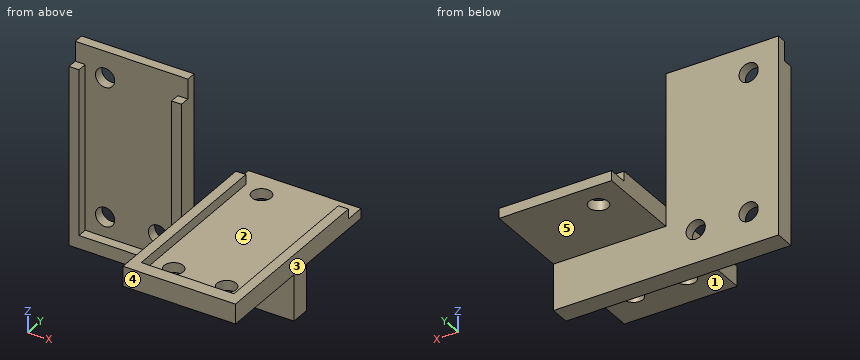
Autodesk Inventor part; units mm, degrees
ref_plane "YZ Plane" through (0, 0, 0) normal (1, 0, 0) x (0, 1, 0)
ref_plane "XZ Plane" through (0, 0, 0) normal (0, 1, 0) x (-1, 0, 0)
ref_plane "XY Plane" through (0, 0, 0) normal (0, 0, 1) x (1, 0, 0)
sketch "Sketch1" plane through (0, 0, 0) normal (0, 0, 1) x (1, 0, 0)
  line L0 (-34, 17) -> (-17, 17)
  line L1 (-17, 17) -> (-17, 30)
  line L2 (-17, 30) -> (0, 30)
  line L3 (0, 30) -> (0, 0)
  line L4 (0, 0) -> (-17, 0)
  line L5 (-17, 0) -> (-17, 14)
  line L6 (-17, 14) -> (-34, 14)
  line L7 (-34, 14) -> (-34, 17)
  dimension "d0" = 17
  dimension "d1" = 13
  dimension "d2" = 17
  dimension "d4" = 17
  dimension "d5" = 14
  dimension "d72" = 3
extrude "Extrusion1" add sketch "Sketch1" along normal blind 30
sketch "Sketch4" plane through (0, 0, 0) normal (0, 0, -1) x (-1, 0, 0)
  line L0 (34, 17) -> (17, 17)
  line L1 (17, 17) -> (17, 30)
  line L2 (17, 30) -> (0, 30)
  line L3 (0, 30) -> (0, 0)
  line L4 (0, 0) -> (17, 0)
  line L5 (17, 0) -> (17, 14)
  line L6 (17, 14) -> (34, 14)
  line L7 (34, 14) -> (34, 17)
  line L8 (17, 0) -> (0, 0)
  line L9 (0, 0) -> (0, 30)
  line L10 (0, 30) -> (17, 30)
  line L11 (17, 30) -> (17, 0)
extrude "Extrusion4" cut sketch "Sketch4" against normal blind 7 contours L11 L5 L4 L3 L2 L1
sketch "Sketch8" plane through (0, 0, 30) normal (0, 0, 1) x (1, 0, 0)
  line L0 (-17, 17) -> (-34, 17)
  line L1 (-34, 17) -> (-34, 14)
  line L2 (-34, 14) -> (-17, 14)
  line L3 (-17, 14) -> (-17, 0)
  line L4 (-17, 0) -> (0, 0)
  line L5 (0, 0) -> (0, 30)
  line L6 (0, 30) -> (-17, 30)
  line L7 (-17, 30) -> (-17, 17)
  line L8 (-17, 30) -> (0, 30)
  line L9 (0, 30) -> (0, 0)
  line L10 (0, 0) -> (-17, 0)
  line L11 (-17, 0) -> (-17, 30)
extrude "Extrusion8" cut sketch "Sketch8" against normal blind 20 contours L7 L6 L5 L4 L3 L11
sketch "Sketch9" plane through (-34, 14, 0) normal (0, -1, 0) x (1, 0, 0)
  line L0 (17, 0) -> (0, 0)
  line L1 (17, 0) -> (17, 7)
  line L2 (17, 7) -> (17, 10)
  line L3 (17, 10) -> (17, 30)
  line L4 (0, 30) -> (17, 30)
  line L5 (0, 0) -> (0, 30)
  line L6 (0, 0) -> (17, 0)
  line L7 (0, 30) -> (17, 30)
  line L8 (17, 0) -> (0, 0)
  line L9 (17, 10) -> (17, 30)
  line L10 (17, 30) -> (0, 30)
  line L11 (0, 0) -> (0, 30)
  line L12 (0, 27) -> (1.5, 27)
  line L13 (1.5, 27) -> (1.5, 2)
  line L14 (1.5, 2) -> (15.5, 2)
  line L15 (17, 27) -> (15.5, 27)
  line L16 (15.5, 27) -> (15.5, 2)
  line L17 (0, 27) -> (0, 30)
  line L18 (17, 30) -> (17, 27)
  point P0 (34, 0)
  dimension "d80" = 1.5
  dimension "d81" = 2
  dimension "d82" = 25
  dimension "d83" = 14
extrude "Extrusion14" cut sketch "Sketch9" against normal blind 1.5 contours L5 L4 L3 L15 L16 L14 L13 L12
sketch "Sketch14" plane through (0, 0, 10) normal (0, 0, 1) x (1, 0, 0)
  line L0 (0, 30) -> (0, 0)
  line L1 (-17, 30) -> (0, 30)
  line L2 (-17, 17) -> (-17, 30)
  line L3 (-17, 14) -> (-17, 17)
  line L4 (-17, 0) -> (-17, 14)
  line L5 (0, 0) -> (-17, 0)
  line L6 (-17, 30) -> (-17, 27)
  line L7 (-17, 30) -> (-17, 17)
  line L8 (-15.5, 27) -> (-15.5, 2)
  line L9 (-15.5, 2) -> (-1.5, 2)
  line L10 (-15.5, 27) -> (-17, 27)
  line L11 (-17, 30) -> (0, 30)
  line L12 (0, 30) -> (-17, 30)
  line L13 (-17, 0) -> (0, 0)
  line L14 (0, 27) -> (0, 30)
  line L15 (-1.5, 27) -> (-1.5, 2)
  line L16 (-1.5, 27) -> (0, 27)
  line L17 (0, 30) -> (0, 0)
  point P0 (0, 30)
  point P1 (-16.25, 27)
  point P2 (-0.75, 27)
  dimension "d87" = 1.5
  dimension "d88" = 2
  dimension "d89" = 25
  dimension "d91" = 1.5
  dimension "d93" = 14
extrude "Extrusion15" cut sketch "Sketch14" against normal blind 1.5 contours L0 L16 L15 L9 L8 L10 L2 L1
sketch "Sketch15" plane through (-34, 15.5, 0) normal (0, -1, 0) x (1, 0, 0)
  line L0 (0, 30) -> (17, 30)
  line L1 (0, 27) -> (0, 30)
  line L2 (1.5, 27) -> (0, 27)
  line L3 (1.5, 2) -> (1.5, 27)
  line L4 (15.5, 2) -> (1.5, 2)
  line L5 (15.5, 27) -> (15.5, 2)
  line L6 (17, 27) -> (15.5, 27)
  line L7 (17, 30) -> (17, 27)
  circle A0 centre (4.5, 26) radius 1.45
  circle A1 centre (4.5, 5) radius 1.45
  circle A2 centre (12.5, 5) radius 1.45
  point P0 (34, 0)
  dimension "d96" = 2.9
  dimension "d97" = 21
  dimension "d98" = 8
  dimension "d99" = 3
  dimension "d100" = 3
extrude "Extrusion16" cut sketch "Sketch15" against normal through all contours A0 | A1 | A2
sketch "Sketch16" plane through (0, 0, 8.5) normal (0, 0, 1) x (1, 0, 0)
  line L0 (-17, 27) -> (-17, 30)
  line L1 (-15.5, 27) -> (-17, 27)
  line L2 (-15.5, 2) -> (-15.5, 27)
  line L3 (-1.5, 2) -> (-15.5, 2)
  line L4 (-1.5, 27) -> (-1.5, 2)
  line L5 (0, 27) -> (-1.5, 27)
  line L6 (0, 30) -> (0, 27)
  line L7 (-17, 30) -> (0, 30)
  circle A0 centre (-12.5, 5) radius 1.45
  circle A1 centre (-4.5, 5) radius 1.45
  circle A2 centre (-12.5, 26) radius 1.45
  point P0 (0, 0)
  dimension "d103" = 3
  dimension "d104" = 3
  dimension "d105" = 8
  dimension "d106" = 21
  dimension "d107" = 2.9
extrude "Extrusion18" cut sketch "Sketch16" against normal through all contours A0 | A1 | A2
sketch "Sketch17" plane through (-17, 14, 0) normal (1, 0, 0) x (0, 0, -1)
  line L0 (0, 0) -> (-7, 0)
  line L1 (0, 3) -> (0, 0)
  line L2 (0, 3) -> (-7, 3)
  line L3 (-7, 3) -> (-7, 0)
  line L4 (0, 0) -> (-7, 0)
  line L5 (-7, 0) -> (-7, 3)
  line L6 (-7, 3) -> (0, 3)
  line L7 (0, 3) -> (0, 0)
  point P0 (0, -14)
  dimension "d54" = 2.7
  dimension "d55" = 21
  dimension "d56" = 3
  dimension "d57" = 8
  dimension "d58" = 3
  dimension "d59" = 2.8
  dimension "d60" = 21
  dimension "d61" = 8
  dimension "d62" = 3
  dimension "d63" = 3
extrude "Extrusion19" add sketch "Sketch17" along normal up to surface (17 mm away) from surface at 0
sketch "Sketch13" plane through (-17, 14, 0) normal (1, 0, 0) x (0, 0, -1)
  line L0 (0, 0) -> (-7, 0)
  line L1 (0, 3) -> (0, 0)
  line L2 (0, 3) -> (-7, 3)
  line L3 (-7, 3) -> (-7, 0)
  line L4 (0, 0) -> (-7, 0)
  line L5 (-7, 0) -> (-7, 3)
  line L6 (-7, 3) -> (0, 3)
  line L7 (0, 3) -> (0, 0)
  point P0 (0, -14)
properties part number "soporte"
Could you check a few things on this model? Use its own coordinates, in mm. Face numbers are marked on the shaded views. A direction names the side the tool comes from. Give positions to 0.01 mm unless a question says otherwise; leave off trailing zeros. Loops run counter-clockwise (first coordinate to the right, second up) from the corner with the lowest first, then second, coordinate; pieces in that order, holes last. Notation, with made-up numbers: (37.25, 29) -> (89.25, 29) arc R30 ccw to (89.25, 64) -> close; hole circle Ø4 at (51, 10.25). An arc over 180 degrees is marked (long way). Answer as CSV lines item,"result". Start each with the question number.
(1) If we section it at C-C on y = 26: Write out the boundary of the cut face in (x, z).
(2) We'd pull the mould along X, two halves only. Please class the marked faces 1, 2 and 3: released by +X, released by -X, zero draft, split by the parting line, or undercut.
(3) I need wall thicknesses on probe 1 along Z at (x, y) = (-29.5, 16.15); probe 2 along X at (y, z) = (14.25, 16.75); probe 3 along Y at (x, z) = (-4.5, 7.65). Which ranges of each line are inside material? Lowest first, please.
(4) I'm going to push flat-ended pins straight in: pin 1 Ø3 at (x, z) = (-27.5, 22) entering from +Y; pin 2 Ø2.5 at (y, z) = (8, 8) entering from -X; pin 3 Ø5 at (x, y) = (-9.5, 17) entering from +Z. Where does each tip first touch, or does it pass through?
(5) If we section it at A-A on y = 4: Write out the boundary of the cut face in (x, z).
(6) If we section it at D-D on z = 5: Write out the boundary of the cut face in (x, y).
(7) If we section it at B-B on x = -5.5: Write out the boundary of the cut face in (y, z), then the cut area to 4 significant figures.
(8) Which directions (+Z, -Z, +X, -X, +Y, -Y) give clear straight access to the entire face, cutting with the end or side of a thin tool? Please do the marked faces 4 and 5.
Computed:
1,outline,"(-17, 7) -> (-13.95, 7) -> (-13.95, 8.5) -> (-15.5, 8.5) -> (-15.5, 10) -> (-17, 10) -> close; (-11.05, 7) -> (0, 7) -> (0, 10) -> (-1.5, 10) -> (-1.5, 8.5) -> (-11.05, 8.5) -> close"
2,face 1,"zero draft"
2,face 2,"undercut"
2,face 3,"released by +X"
3,probe 1,"z = 0 to 3.55, 6.45 to 24.55, 27.45 to 30"
3,probe 2,"x = -34 to -32.5, -18.5 to -17"
3,probe 3,"y = 0 to 3.55, 6.45 to 30"
4,pin 1,"stops at y = 17"
4,pin 2,"stops at x = -17"
4,pin 3,"stops at z = 8.5"
5,outline,"(-17, 7) -> (-13.55, 7) -> (-13.55, 8.5) -> (-15.5, 8.5) -> (-15.5, 10) -> (-17, 10) -> close; (-11.45, 7) -> (-5.55, 7) -> (-5.55, 8.5) -> (-11.45, 8.5) -> close; (-3.45, 7) -> (0, 7) -> (0, 10) -> (-1.5, 10) -> (-1.5, 8.5) -> (-3.45, 8.5) -> close"
6,outline,"(-34, 14) -> (-32.5, 14) -> (-32.5, 15.5) -> (-30.95, 15.5) -> (-30.95, 17) -> (-34, 17) -> close; (-28.05, 15.5) -> (-22.95, 15.5) -> (-22.95, 17) -> (-28.05, 17) -> close; (-20.05, 15.5) -> (-18.5, 15.5) -> (-18.5, 14) -> (0, 14) -> (0, 17) -> (-20.05, 17) -> close"
7,outline,"(0, 7) -> (3.95, 7) -> (3.95, 8.5) -> (2, 8.5) -> (2, 10) -> (0, 10) -> close; (6.05, 7) -> (14, 7) -> (14, 0) -> (17, 0) -> (17, 7) -> (30, 7) -> (30, 8.5) -> (6.05, 8.5) -> close"
7,area,"65.85 mm2"
8,face 4,"+Z, -Z, +X, -X, -Y"
8,face 5,"-Z, +X, -X, +Y"
